Part model, mm, in its own coordinate system. A direction names the side the tool comes from. Round coordinates to 2 decimals unless told otherwise and drop trailing zeros. Loops run counter-clockwise (first coordinate to the right, second up) from the corner with the lowest first, then second, coordinate; pieces in that order, holes last.
from build123d import *

# Parameters (mm, degrees)
BOSS_EXTRUDE1_REACH      = 1519.328
BOSS_EXTRUDE1_END_RADIUS = 400
BOSS_EXTRUDE2_REACH      = 1605.109
BOSS_EXTRUDE2_END_RADIUS = 400
SKETCH5_W                = 50.8
SKETCH5_H                = 50.8


with BuildPart() as part:
    # Sketch1 → Revolve1 (revolve)
    with BuildSketch(Plane.XY):
        with BuildLine():
            Line((150, -400), (1050, -400))
            ThreePointArc((1050, -400), (1154.808037789, -230.089635957), (1198.969132037, -35.4))
            Line((1198.969132037, -35.4), (1224.369132037, -35.4))
            Line((1224.369132037, -35.4), (1224.369132037, -25.4))
            Line((1224.369132037, -25.4), (1199.469500194, -25.4))
            Line((1199.469500194, -25.4), (1189.460625969, -25.4))
            ThreePointArc((1189.460625969, -25.4), (1148.153333745, -219.830314428), (1045.431779669, -390))
            Line((1045.431779669, -390), (154.568220331, -390))
            ThreePointArc((154.568220331, -390), (47.305004997, -207.966325597), (10, 0))
            Line((10, 0), (0, 0))
            ThreePointArc((0, 0), (38.733083645, -213.600093633), (150, -400))
        make_face()
    revolve(axis=Axis((0, 0, 0), (1, 0, 0)))

    # Boss-Extrude1: up to this cylinder (the profile starts outside it)
    boss_extrude1_end = Plane(origin=(1028.779341, 0, 0), z_dir=(-1, 0, 0)) * Cylinder(BOSS_EXTRUDE1_END_RADIUS, 3839.656, mode=Mode.PRIVATE)
    # Sketch4 → Boss-Extrude1 (add, up to the surface)
    with BuildSketch(Plane(origin=(0, 0, -402), x_dir=(-1, 0, 0), z_dir=(0, 0, -1)), mode=Mode.PRIVATE) as boss_extrude1_sk1:
        with BuildLine():
            Line((-1050, 173.312071556), (-1050, 273.312071556))
            ThreePointArc((-1050, 273.312071556), (-1000, 223.312071556), (-1050, 173.312071556))
        make_face()
    boss_extrude1_tool1 = extrude(boss_extrude1_sk1.sketch, amount=-BOSS_EXTRUDE1_REACH, mode=Mode.PRIVATE) - boss_extrude1_end
    add(boss_extrude1_tool1.solids().sort_by_distance((1028.779341, 223.312072, -402))[0])
    # Sketch4 → Boss-Extrude1 (add, up to the surface)
    with BuildSketch(Plane(origin=(0, 0, -402), x_dir=(-1, 0, 0), z_dir=(0, 0, -1)), mode=Mode.PRIVATE) as boss_extrude1_sk2:
        with BuildLine():
            Line((-1050, -173.312071556), (-1050, -273.312071556))
            ThreePointArc((-1050, -273.312071556), (-1000, -223.312071556), (-1050, -173.312071556))
        make_face()
    boss_extrude1_tool2 = extrude(boss_extrude1_sk2.sketch, amount=-BOSS_EXTRUDE1_REACH, mode=Mode.PRIVATE) - boss_extrude1_end
    add(boss_extrude1_tool2.solids().sort_by_distance((1028.779341, -223.312072, -402))[0])

    # Boss-Extrude2: up to this cylinder (the profile starts outside it)
    boss_extrude2_end = Plane(origin=(600, 0, 0), z_dir=(-1, 0, 0)) * Cylinder(BOSS_EXTRUDE2_END_RADIUS, 4860.418, mode=Mode.PRIVATE)
    # Sketch5 → Boss-Extrude2 (add, up to the surface)
    with BuildSketch(Plane.XY.offset(552.4), mode=Mode.PRIVATE) as boss_extrude2_sk1:
        with Locations((1024.6, 177.8)):
            Rectangle(SKETCH5_W, SKETCH5_H)
    boss_extrude2_tool1 = extrude(boss_extrude2_sk1.sketch, amount=-BOSS_EXTRUDE2_REACH, mode=Mode.PRIVATE) - boss_extrude2_end
    add(boss_extrude2_tool1.solids().sort_by_distance((1024.6, 177.8, 552.4))[0])
    # Sketch5 → Boss-Extrude2 (add, up to the surface)
    with BuildSketch(Plane.XY.offset(552.4), mode=Mode.PRIVATE) as boss_extrude2_sk2:
        with Locations((175.4, 177.8)):
            Rectangle(SKETCH5_W, SKETCH5_H)
    boss_extrude2_tool2 = extrude(boss_extrude2_sk2.sketch, amount=-BOSS_EXTRUDE2_REACH, mode=Mode.PRIVATE) - boss_extrude2_end
    add(boss_extrude2_tool2.solids().sort_by_distance((175.4, 177.8, 552.4))[0])
    # Sketch5 → Boss-Extrude2 (add, up to the surface)
    with BuildSketch(Plane.XY.offset(552.4), mode=Mode.PRIVATE) as boss_extrude2_sk3:
        with Locations((1024.6, -127)):
            Rectangle(SKETCH5_W, SKETCH5_H)
    boss_extrude2_tool3 = extrude(boss_extrude2_sk3.sketch, amount=-BOSS_EXTRUDE2_REACH, mode=Mode.PRIVATE) - boss_extrude2_end
    add(boss_extrude2_tool3.solids().sort_by_distance((1024.6, -127, 552.4))[0])
    # Sketch5 → Boss-Extrude2 (add, up to the surface)
    with BuildSketch(Plane.XY.offset(552.4), mode=Mode.PRIVATE) as boss_extrude2_sk4:
        with Locations((175.4, -127)):
            Rectangle(SKETCH5_W, SKETCH5_H)
    boss_extrude2_tool4 = extrude(boss_extrude2_sk4.sketch, amount=-BOSS_EXTRUDE2_REACH, mode=Mode.PRIVATE) - boss_extrude2_end
    add(boss_extrude2_tool4.solids().sort_by_distance((175.4, -127, 552.4))[0])


solid = part.part
1) Tool access for faces 5 (the face through (150, 177, 450)), 6 (the face through (1050, -234, -360)), 7 (the face through (1211.847, -33.765, -10.633)): list every direction of +Z, -Z, +X, -X, +Y, -Y with a clear straight run to the whole face (end or side of a thin tool).
Values:
face 5: +Z, -X, +Y
face 6: -Z, +X, -Y
face 7: +X
2) Mould opens along Y. For faces 1 (the face through (1024, 203.2, 450)), 2 (the face through (175, 152.4, 462)), 3 (the face through (1050, -127, 462)), 4 (the face through (1024, -101.6, 471)) say: released by +Y, released by -Y, zero draft, split by the parting line, or undercut.
Values:
face 1: released by +Y
face 2: undercut
face 3: zero draft
face 4: undercut
3) Slice it at C-C, the plane x = 301. Give the cut face in (y, z), then the cut area to 3 significant figures.
Values:
outline: circle Ø800 at (0, 0); hole circle Ø780 at (0, 0)
area: 24,800 mm2
4) Drop flat-ended pins along their axis: pin 1 Ø6 at (y, z) = (-305.5, 220) entering from +X; pin 2 Ø5 at (x, z) = (729, -73) entering from -Y; pin 3 Ø3 at (x, y) = (904.5, 220.5) entering from -Z. Give the stop position or say it passes through.
Values:
pin 1: stops at x = 1071.86
pin 2: stops at y = -393.74
pin 3: stops at z = -334.72
5) Slice it at A-A, the plane z = -317. Give the cut face in (x, y).
Values:
outline: (150, -243.95) - (1004.46, -243.95) arc R50 ccw to (1050, -273.31) - (1050, -243.95) arc R519.21 ccw to (1050, 243.95) - (1050, 273.31) arc R50 ccw to (1004.46, 243.95) - (150, 243.95) arc R519.21 ccw to start; hole (154.57, -227.18) - (1045.43, -227.18) arc R507.46 ccw to (1045.43, 227.18) - (154.57, 227.18) arc R507.46 ccw to start
6) Slice it at D-D, the plane z = 0. Give the cut face in (x, y).
Values:
outline: (150, -400) - (1050, -400) arc R608.33 ccw to (1198.97, -35.4) - (1224.37, -35.4) - (1224.37, -25.4) - (1189.46, -25.4) arc R598.33 cw to (1045.43, -390) - (154.57, -390) arc R598.33 cw to (154.57, 390) - (1045.43, 390) arc R598.33 cw to (1189.46, 25.4) - (1224.37, 25.4) - (1224.37, 35.4) - (1198.97, 35.4) arc R608.33 ccw to (1050, 400) - (150, 400) arc R608.33 ccw to start
7) Wall check: line 1 along Y through (x, z) = (1202, 0); line 2 along Y through (x, z) = (534, 0). Give the ranges that are in metal, low to high.
Values:
line 1: y = -35.4 to -25.4, 25.4 to 35.4
line 2: y = -400 to -390, 390 to 400
8) Slice it at B-B, the plane y = -118.5. Give the cut face in (x, z), then the cut area to 3 significant figures.
Values:
outline: (150, -382.04) - (1050, -382.04) arc R596.68 ccw to (1050, 382.04) - (1050, 552.4) - (999.2, 552.4) - (999.2, 382.04) - (200.8, 382.04) - (200.8, 552.4) - (150, 552.4) - (150, 382.04) arc R596.68 ccw to start; hole (154.57, -371.56) - (1045.43, -371.56) arc R586.48 ccw to (1045.43, 371.56) - (154.57, 371.56) arc R586.48 ccw to start
area: 52,700 mm2
